```python
from build123d import *

# Parameters (mm, degrees)
SKETCH1_W           = 23
SKETCH1_H           = 20
BOSS_EXTRUDE1_DEPTH = 3
BOSS_EXTRUDE2_DEPTH = 20
CUT_EXTRUDE2_DEPTH  = 2
LPATTERN2_COUNT     = 2
LPATTERN2_PITCH     = 10
SKETCH6_R           = 2.5
CUT_EXTRUDE3_DEPTH  = 4
SKETCH7_W           = 15.359271736
SKETCH7_H           = 20
CUT_EXTRUDE4_DEPTH  = 1


with BuildPart() as part:
    # Sketch1 → Boss-Extrude1 (new body)
    with BuildSketch(Plane.XY):
        with Locations((0.940520446, -4.763011152)):
            Rectangle(SKETCH1_W, SKETCH1_H)
    extrude(amount=BOSS_EXTRUDE1_DEPTH)

    # Sketch2 → Boss-Extrude2 (add, through all)
    with BuildSketch(Plane(origin=(0, 5.236988848, 0), x_dir=(1, 0, 0), z_dir=(0, 1, 0))):
        with BuildLine():
            ThreePointArc((1.417746021, -3), (-0.936980555, -0.799122875), (-4.059479554, 0))
            Line((-4.059479554, 0), (-4.059479554, -3))
            Line((-4.059479554, -3), (1.417746021, -3))
        make_face()
        with BuildLine():
            Line((-4.059479554, -3), (-4.059479554, 0))
            ThreePointArc((-4.059479554, 0), (-7.181978553, -0.799122875), (-9.536705129, -3))
            Line((-9.536705129, -3), (-4.059479554, -3))
        make_face()
        with BuildLine():
            Line((1.417746021, -3), (-4.059479554, -3))
            Line((-4.059479554, -3), (-4.059479554, -4))
            ThreePointArc((-4.059479554, -4), (-2.291712601, -4.732233047), (-1.559479554, -6.5))
            ThreePointArc((-1.559479554, -6.5), (-2.291712601, -8.267766953), (-4.059479554, -9))
            Line((-4.059479554, -9), (-4.059479554, -13))
            ThreePointArc((-4.059479554, -13), (0.536714524, -11.096194078), (2.440520446, -6.5))
            ThreePointArc((2.440520446, -6.5), (2.179589537, -4.676811342), (1.417746021, -3))
        make_face()
        with BuildLine():
            Line((-4.059479554, -4), (-4.059479554, -3))
            Line((-4.059479554, -3), (-9.536705129, -3))
            ThreePointArc((-9.536705129, -3), (-10.298548645, -4.676811342), (-10.559479554, -6.5))
            ThreePointArc((-10.559479554, -6.5), (-8.655673632, -11.096194078), (-4.059479554, -13))
            Line((-4.059479554, -13), (-4.059479554, -9))
            ThreePointArc((-4.059479554, -9), (-6.559479554, -6.5), (-4.059479554, -4))
        make_face()
        with BuildLine():
            ThreePointArc((-10.559479554, -6.5), (-10.298548645, -4.676811342), (-9.536705129, -3))
            Line((-9.536705129, -3), (-10.559479554, -3))
            Line((-10.559479554, -3), (-10.559479554, -6.5))
        make_face()
        with BuildLine():
            Line((2.440520446, -3), (1.417746021, -3))
            ThreePointArc((1.417746021, -3), (2.179589537, -4.676811342), (2.440520446, -6.5))
            Line((2.440520446, -6.5), (2.440520446, -3))
        make_face()
    extrude(amount=-BOSS_EXTRUDE2_DEPTH)

    # Sketch4 → Cut-Extrude2 (cut, symmetric)
    with BuildSketch(Plane(origin=(0, 0.236988848, 0), x_dir=(-1, 0, 0), z_dir=(0, -1, 0))):
        Polygon((0.059479554, -2.5), (8.059479554, -2.5), (8.059479554, -10.5), (8.059479554, -14.57083766), (0.059479554, -14.57083766), (0.059479554, -10.5), align=None)
    cut_extrude2 = extrude(amount=CUT_EXTRUDE2_DEPTH, both=True, mode=Mode.SUBTRACT)

    # LPattern2: Cut-Extrude2 ×2
    with Locations(*[(0, -i * LPATTERN2_PITCH, 0) for i in range(1, LPATTERN2_COUNT)]):
        add(cut_extrude2, mode=Mode.SUBTRACT)

    # Sketch6 → Cut-Extrude3 (cut)
    with BuildSketch(Plane.XY.offset(3)):
        with Locations((7.440520446, -4.763011152)):
            Circle(SKETCH6_R)
    extrude(amount=-CUT_EXTRUDE3_DEPTH, mode=Mode.SUBTRACT)

    # Sketch7 → Cut-Extrude4 (cut)
    with BuildSketch(Plane.ZY.offset(10.559479554)):
        with Locations((7.679635868, -4.763011152)):
            Rectangle(SKETCH7_W, SKETCH7_H)
    extrude(amount=-CUT_EXTRUDE4_DEPTH, mode=Mode.SUBTRACT)


solid = part.part
```
The listing builds one solid part. Answer for the finished solid, in the listing's coordinates (mm). A direction names the side the tool comes from. Round coordinates to 2 decimals unless told otherwise and drop trailing zeros. Loops run counter-clockwise (first coordinate to the right, second up) from the corner with the lowest first, then second, coordinate; pieces in that order, holes last.
1) Consider line 1 (Y direction, x = -7.25, z = 6.5); line 2 (X direction, y = -0.25, z = 4); line 3 (X direction, y = -10.75, z = 10). Determine where each line is inside the solid, lowest interval first.
Outcome:
line 1: y = -14.76 to -11.76, -7.76 to -1.76, 2.24 to 5.24
line 2: x = -9.56 to -8.06, -0.06 to 2.44
line 3: x = -9.54 to -8.06, -0.06 to 1.42
2) For a pull along Y with two mould halves and no side action, classify faces 4 (the face through (6, -2, 3)), 5 (the face through (-0.059, -10, 7)), 6 (the face through (-1, -14.763, 5)) as released by +Y, released by -Y, zero draft, split by the parting line, or undercut.
Outcome:
face 4: zero draft
face 5: undercut
face 6: released by -Y
3) A cutting plane is placed at B-B on z = 12. Determine the outline of the cut face in (x, y).
Outcome:
outline: (-7.52, -14.76) - (-0.6, -14.76) - (-0.6, -11.76) - (-7.52, -11.76) - close; (-7.52, -7.76) - (-0.6, -7.76) - (-0.6, -1.76) - (-7.52, -1.76) - close; (-7.52, 2.24) - (-0.6, 2.24) - (-0.6, 5.24) - (-7.52, 5.24) - close
4) A cutting plane is placed at D-D on x = 2.75. Determine the outline of the cut face in (y, z).
Outcome:
outline: (-14.76, 0) - (5.24, 0) - (5.24, 3) - (-14.76, 3) - close
5) For faces 1 (the face through (-5, 2.237, 9)), 2 (the face through (-9.559, -5, 5)), 3 (the face through (2.441, -5, 5)), determine the directions among +Z, -Z, +X, -X, +Y, -Y from which every point of the face is accessible in a straight line to the end or side of a thin tool.
Outcome:
face 1: +Z
face 2: +Z, -Z, -X, +Y, -Y
face 3: +Z, +X, +Y, -Y
6) Given P1, Ø3, axis at x = -7.5, y = 0.5, coming from the +Z side; P2, Ø3, axis at y = 1, z = 8.5, coming from the +X side; P3, Ø3, axis at x = -5, y = -9.5, coming from the +Z side, each flat-ended and moving along its own axis, determine where each tip first touches the part or whether it passes through.
Outcome:
P1: stops at z = 11.62
P2: stops at x = 2.42
P3: stops at z = 2.5
7) A cutting plane is placed at C-C on z = 6. Determine the outline of the cut face in (x, y).
Outcome:
outline: (-9.56, -14.76) - (-6.51, -14.76) - (-6.51, -11.76) - (-8.06, -11.76) - (-8.06, -7.76) - (-6.51, -7.76) - (-6.51, -1.76) - (-8.06, -1.76) - (-8.06, 2.24) - (-6.51, 2.24) - (-6.51, 5.24) - (-9.56, 5.24) - close; (-1.61, -14.76) - (2.44, -14.76) - (2.44, 5.24) - (-1.61, 5.24) - (-1.61, 2.24) - (-0.06, 2.24) - (-0.06, -1.76) - (-1.61, -1.76) - (-1.61, -7.76) - (-0.06, -7.76) - (-0.06, -11.76) - (-1.61, -11.76) - close
8) A cutting plane is placed at A-A on y = -1.5. Determine the outline of the cut face in (x, z), plus the area to 3 significant figures.
Outcome:
outline: (-9.56, 0) - (12.44, 0) - (12.44, 3) - (2.44, 3) - (2.44, 6.5) arc R6.5 ccw to (-0.06, 11.62) - (-0.06, 2.5) - (-8.06, 2.5) - (-8.06, 11.62) arc R6.5 ccw to (-9.56, 9.96) - close
area: 91.5 mm2
